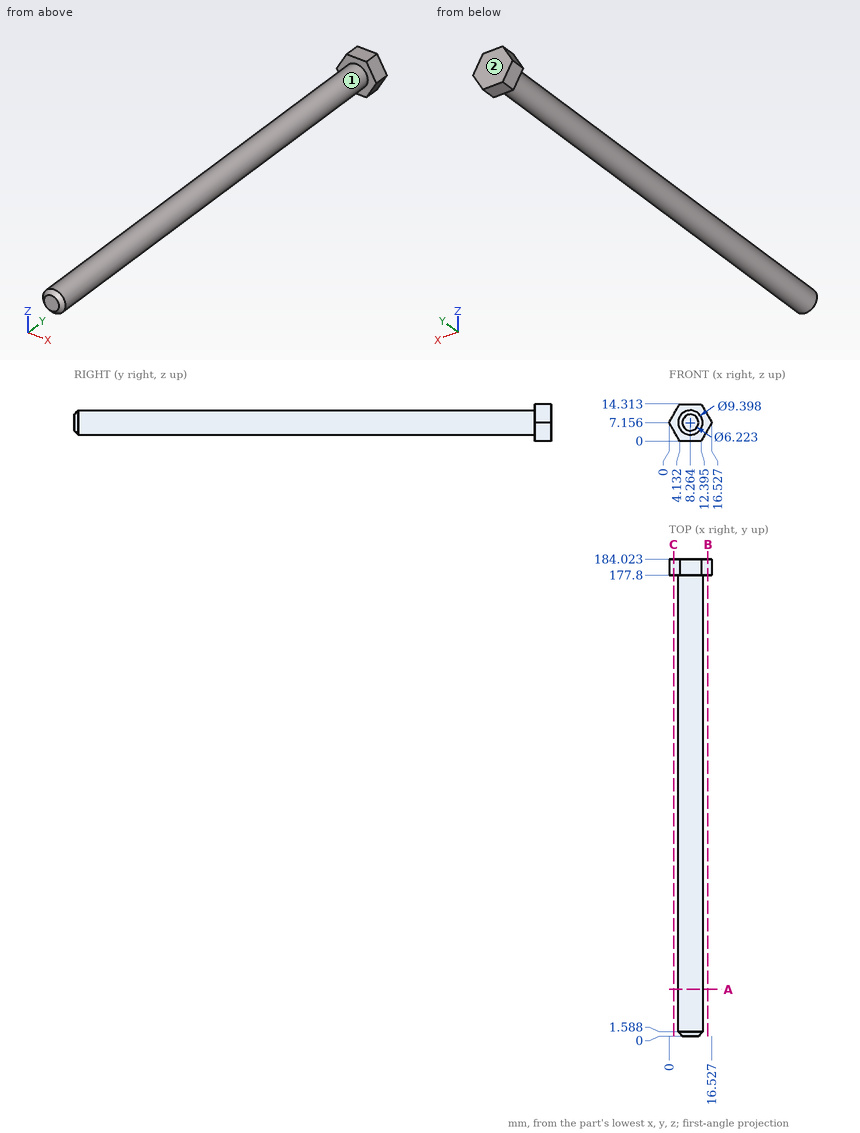
Answer from the drawing. Dimensions are ordinates in mm from the lowest x, y and z of the part. A direction names the side the tool comes from. Round coordinates to 2 decimals unless told otherwise and drop trailing zeros. Loops run counter-clockwise (first coordinate to the right, second up) from the corner with the lowest first, then second, coordinate; pieces in that order, holes last.
Q1. Consider probe 1 along Y at (x, z) = (7, 13); probe 2 along Z at (x, y) = (8.25, 29.5) (1 decimal); probe 3 along X at (y, z) = (37.5, 10.25) (1 decimal). Determine where each line is inside the solid, lowest interval first.
Q2. Section B-B on x = 15 is taken. Write down the section's boundary in (y, z), and give its area (3 significant figures).
Q3. Section C-C on x = 1.75 is taken. Write down the section's boundary in (y, z) (1 decimal), and give its area (3 significant figures).
Q4. Section A-A on y = 18 is taken. Write down the section's boundary in (x, z).
Q5. Which of the six approach directions +Z, -Z, +X, -X, +Y, -Y give full straight-line access (tool end or side, diameter ignored) to the marked faces 1 and 2?
Q6. Each of these flat-tipped pins is pushed along its axis until it touches: pin 1 (6 mm diameter, centred on x = 6.5, y = 135, fed in from -Z); pin 2 (1.5 mm diameter, centred on x = 8, y = 127, fed in from +Z) (1 decimal); pin 3 (3 mm diameter, centred on x = 11, y = 70, fed in from -Z). Where does it stop, or does it pass through?
Output:
1. probe 1: y = 177.8 to 184.02
1. probe 2: z = 2.5 to 11.9
1. probe 3: x = 4.7 to 11.8
2. outline: (177.8, 4.51) - (184.02, 4.51) - (184.02, 9.8) - (177.8, 9.8) - close
2. area: 32.9 mm2
3. outline: (177.8, 4.1) - (184, 4.1) - (184, 10.2) - (177.8, 10.2) - close
3. area: 37.7 mm2
4. outline: circle Ø9.4 at (8.26, 7.16)
5. face 1: -Y
5. face 2: +Z, -Z, +X, -X, +Y
6. pin 1: stops at z = 2.46
6. pin 2: stops at z = 11.9
6. pin 3: stops at z = 2.62
